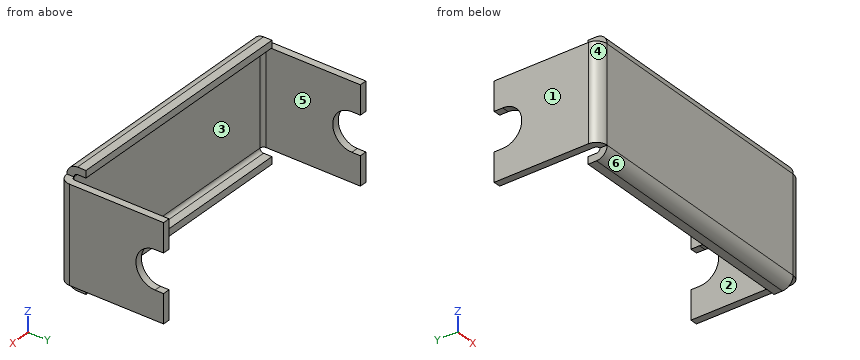
```python
from build123d import *

# Parameters (mm, degrees)
CROQUIS3_W                         = 55.5
CROQUIS3_H                         = 20
BRIDA_BASE1_DEPTH                  = 1.5
BRIDA_DE_ARISTA1_STRIP_W           = 7.4732
BRIDA_DE_ARISTA1_STRIP_H           = 1.5
BRIDA_DE_ARISTA1_STRIP_CUT_DEPTH   = 20
BRIDA_DE_ARISTA1_STRIP_2_W         = 7.4732
BRIDA_DE_ARISTA1_STRIP_2_H         = 1.5
BRIDA_DE_ARISTA1_STRIP_CUT_2_DEPTH = 20
BRIDA_DE_ARISTA1_DEPTH             = 20
BRIDA_DE_ARISTA1_BEND_DEPTH        = 20
BRIDA_DE_ARISTA2_DEPTH             = 51.0268
BRIDA_DE_ARISTA2_BEND_DEPTH        = 51.0268
CORTAR_EXTRUIR1_REACH              = 62.417


# Sheet-metal steps are written as plain solids
with BuildPart() as part:
    # Croquis3 → Brida base1 (new body)
    with BuildSketch(Plane(origin=(0, 0, 0), x_dir=(1, 0, 0), z_dir=(0, 1, 0))):
        Rectangle(CROQUIS3_W, CROQUIS3_H)
    extrude(amount=-BRIDA_BASE1_DEPTH)

    # Brida de arista1 strip (across the edge) → Brida de arista1 strip cut (cut)
    with BuildSketch(Plane(origin=(-27.75, 0, -10), x_dir=(1, 0, 0), z_dir=(0, 0, 1))):
        with Locations((-1.5, -0.75)):
            Rectangle(BRIDA_DE_ARISTA1_STRIP_W, BRIDA_DE_ARISTA1_STRIP_H)
    extrude(amount=BRIDA_DE_ARISTA1_STRIP_CUT_DEPTH, mode=Mode.SUBTRACT)

    # Brida de arista1 strip 2 (across the edge) → Brida de arista1 strip cut 2 (cut)
    with BuildSketch(Plane(origin=(27.75, 0, 10), x_dir=(-1, 0, 0), z_dir=(0, 0, -1))):
        with Locations((-1.5, -0.75)):
            Rectangle(BRIDA_DE_ARISTA1_STRIP_2_W, BRIDA_DE_ARISTA1_STRIP_2_H)
    extrude(amount=BRIDA_DE_ARISTA1_STRIP_CUT_2_DEPTH, mode=Mode.SUBTRACT)

    # Brida de arista1 section (across the edge) → Brida de arista1 (add)
    with BuildSketch(Plane(origin=(-27.75, 0, -10), x_dir=(1, 0, 0), z_dir=(0, 0, 1))):
        with BuildLine():
            Line((0, 0.7366), (0, 20.5))
            Line((0, 20.5), (1.5, 20.5))
            Line((1.5, 20.5), (1.5, 0.7366))
            ThreePointArc((1.5, 0.7366), (1.715745145, 0.215745145), (2.2366, 0))
            Line((2.2366, 0), (2.2366, -1.5))
            ThreePointArc((2.2366, -1.5), (0.655084973, -0.844915027), (0, 0.7366))
        make_face()
    extrude(amount=BRIDA_DE_ARISTA1_DEPTH)

    # Brida de arista1 section 2 (across the edge) → Brida de arista1 bend (add)
    with BuildSketch(Plane(origin=(27.75, 0, 10), x_dir=(-1, 0, 0), z_dir=(0, 0, -1))):
        with BuildLine():
            Line((0, 0.7366), (0, 20.5))
            Line((0, 20.5), (1.5, 20.5))
            Line((1.5, 20.5), (1.5, 0.7366))
            ThreePointArc((1.5, 0.7366), (1.715745145, 0.215745145), (2.2366, 0))
            Line((2.2366, 0), (2.2366, -1.5))
            ThreePointArc((2.2366, -1.5), (0.655084973, -0.844915027), (0, 0.7366))
        make_face()
    extrude(amount=BRIDA_DE_ARISTA1_BEND_DEPTH)

    # Brida de arista2 section (across the edge) → Brida de arista2 (add)
    with BuildSketch(Plane(origin=(-25.5134, 0, 10.7366), x_dir=(0, 0, -1), z_dir=(1, 0, 0))):
        with BuildLine():
            Line((-1.5, 0.7366), (-1.5, 2.5))
            Line((-1.5, 2.5), (0, 2.5))
            Line((0, 2.5), (0, 0.7366))
            ThreePointArc((0, 0.7366), (0.215745145, 0.215745145), (0.7366, 0))
            Line((0.7366, 0), (0.7366, -1.5))
            ThreePointArc((0.7366, -1.5), (-0.844915027, -0.844915027), (-1.5, 0.7366))
        make_face()
    extrude(amount=BRIDA_DE_ARISTA2_DEPTH)

    # Brida de arista2 section 2 (across the edge) → Brida de arista2 bend (add)
    with BuildSketch(Plane(origin=(25.5134, 0, -10.7366), x_dir=(0, 0, 1), z_dir=(-1, 0, 0))):
        with BuildLine():
            Line((-1.5, 0.7366), (-1.5, 2.5))
            Line((-1.5, 2.5), (0, 2.5))
            Line((0, 2.5), (0, 0.7366))
            ThreePointArc((0, 0.7366), (0.215745145, 0.215745145), (0.7366, 0))
            Line((0.7366, 0), (0.7366, -1.5))
            ThreePointArc((0.7366, -1.5), (-0.844915027, -0.844915027), (-1.5, 0.7366))
        make_face()
    extrude(amount=BRIDA_DE_ARISTA2_BEND_DEPTH)

    # Cortar-Extruir1: up to this face of the body (flat: up to its plane)
    cortar_extruir1_end = Plane(part.part.faces().sort_by_distance((-27.75, 10.6183, 0))[0])
    # Croquis20 → Cortar-Extruir1 (cut, up to the picked face)
    with BuildSketch(Plane(origin=(27.75, 0, 0), x_dir=(0, 0, -1), z_dir=(1, 0, 0)), mode=Mode.PRIVATE) as cortar_extruir1_sk1:
        with BuildLine():
            Line((4, 18.7), (4, 22.7))
            Line((4, 22.7), (-4, 22.7))
            Line((-4, 22.7), (-4, 18.7))
            ThreePointArc((-4, 18.7), (0, 14.7), (4, 18.7))
        make_face()
    cortar_extruir1_tool1 = split(extrude(cortar_extruir1_sk1.sketch, amount=-CORTAR_EXTRUIR1_REACH, mode=Mode.PRIVATE), bisect_by=cortar_extruir1_end, keep=Keep.BOTH, mode=Mode.PRIVATE)
    add(cortar_extruir1_tool1.solids().sort_by(Axis((27.75, 19.073399, 0), (-1, 0, 0)))[0], mode=Mode.SUBTRACT)


solid = part.part
```
The listing builds one solid part. Answer for the finished solid, in the listing's coordinates (mm). Face numbers are marked on the shaded views. A direction names the side the tool comes from. Coordinates: 2 decimals unless noted, no trailing zeros. Loops run counter-clockwise (first coordinate to the right, second up) from the corner with the lowest first, then second, coordinate; pieces in that order, holes last. Notation, with made-up numbers: M 38.25,-23.75 L 86.25,-23.75 A28 cw 86.25,3.25 Z; hole C 32,37 d4. An arc over 180 degrees is marked long. Answer as a JSON object with one key per item and string values. Group by question number.
Item 1: Consider L1, parallel to X at y = 16.25, z = 7.75; L2, parallel to Z at x = 24.5, y = 2; L3, parallel to Y at x = -16, z = -4.25. Determine where each line is inside the solid, lowest interval first.
Item 2: Determine the mould class of the marked faces 4, 5 and 6 for opening direction X: +X half, -X half, draft (parallel to the pull), parting line (faces both ways), or undercut.
Item 3: Which of the six approach directions +Z, -Z, +X, -X, +Y, -Y give full straight-line access (tool end or side, diameter ignored) to the marked faces 1, 2 and 3?
Item 4: Section B-B (z = 0) is taken. Write down the section's boundary in (x, y), and give its area (3 significant figures).
Item 5: Section A-A (y = 10.75) is taken. Write down the section's boundary in (x, z), and give its area (3 significant figures).
Item 6: Section C-C (x = 15) is taken. Write down the section's boundary in (y, z).
Item 7: Each of these flat-tipped pins is pushed along its axis until it touches: P1, Ø10, axis at x = 16.5, z = -7.5, coming from the +Y side; P2, Ø0.8, axis at x = -27, y = 19.5, coming from the +Z side; P3, Ø1.1, axis at y = 0.5, z = 10.5, coming from the -X side; P4, Ø1.8, axis at y = 1, z = -11, coming from the +X side. Where does it stop, or does it pass through?
Solved:
{
 "1": {"L1": "x = -27.75 to -26.25, 26.25 to 27.75", "L2": "z = -12.24 to -10.74, 10.74 to 12.24", "L3": "y = -1.5 to 0"},
 "2": {"face 4": "-X half", "face 5": "undercut", "face 6": "draft"},
 "3": {"face 1": "+Z, -Z, -X, +Y, -Y", "face 2": "+Z, -Z, +Y", "face 3": "+Y"},
 "4": {"outline": "M -27.75,0.74 A2.24 ccw -25.51,-1.5 L 25.51,-1.5 A2.24 ccw 27.75,0.74 L 27.75,14.7 L 26.25,14.7 L 26.25,0.74 A0.74 cw 25.51,0 L -25.51,0 A0.74 cw -26.25,0.74 L -26.25,14.7 L -27.75,14.7 Z", "area": "125 mm2"},
 "5": {"outline": "M -27.75,-10 L -26.25,-10 L -26.25,10 L -27.75,10 Z; M 26.25,-10 L 27.75,-10 L 27.75,10 L 26.25,10 Z", "area": "60.0 mm2"},
 "6": {"outline": "M -1.5,-10 A2.24 ccw 0.74,-12.24 L 2.5,-12.24 L 2.5,-10.74 L 0.74,-10.74 A0.74 cw 0,-10 L 0,10 A0.74 cw 0.74,10.74 L 2.5,10.74 L 2.5,12.24 L 0.74,12.24 A2.24 ccw -1.5,10 Z"},
 "7": {"P1": "stops at y = 2.5", "P2": "stops at z = 10", "P3": "stops at x = -27.75", "P4": "stops at x = 25.51"}
}
